The drawing under review shows one solid part. Ordinate dimensions are in mm from its lowest x, y, z. A direction names the side the tool comes from. Coordinates: 2 decimals unless noted, no trailing zeros. Loops run counter-clockwise (first coordinate to the right, second up) from the corner with the lowest first, then second, coordinate; pieces in that order, holes last. Notation, with made-up numbers: (57.25, -9) - (79.25, -9) arc R11 cw to (79.25, -4) - close; hole circle Ø6 at (86.25, 13). An arc over 180 degrees is marked (long way). Answer as a JSON object with one key per item and string values. Group by question number.
Item 1: We need section B-B (z = 12.75). Give the boundary of the cut face in (x, y).
Item 2: We need section A-A (x = 14.25). Give the boundary of the cut face in (y, z), then the cut area to 3 significant figures.
Item 3: We need section C-C (y = 44). Give the boundary of the cut face in (x, z), then the cut area to 3 significant figures.
Item 4: Tool access review of the marked faces 1, 2, 3 and 4: name each direction out of +Z, -Z, +X, -X, +Y, -Y from which nothing blocks a thin tool from reaching the whole face with its end or side.
Item 5: To check wall thickness, follow line 1 (Y direction, x = 2, z = 23); line 2 (Z direction, x = 6.5, y = 6.5); line 3 (Z direction, x = 6, y = 65.5). State the ranges of each line that lie inside material, in increasing order.
Item 6: We need section D-D (z = 6.25). Give the boundary of the cut face in (x, y).
Item 7: Clearance check with flat-ended pins moving along their axes: pin 1 (10 mm diameter, centred on x = 16.5, y = 45.5, fed in from -Z); pin 2 (7.5 mm diameter, centred on y = 42, z = 18, fed in from -X); pin 3 (7.5 mm diameter, centred on y = 42.5, z = 16.5, fed in from +X); pin 4 (5 mm diameter, centred on x = 21.5, y = 53.5, fed in from +Z). State where each tip first meets the part, or that it passes through.
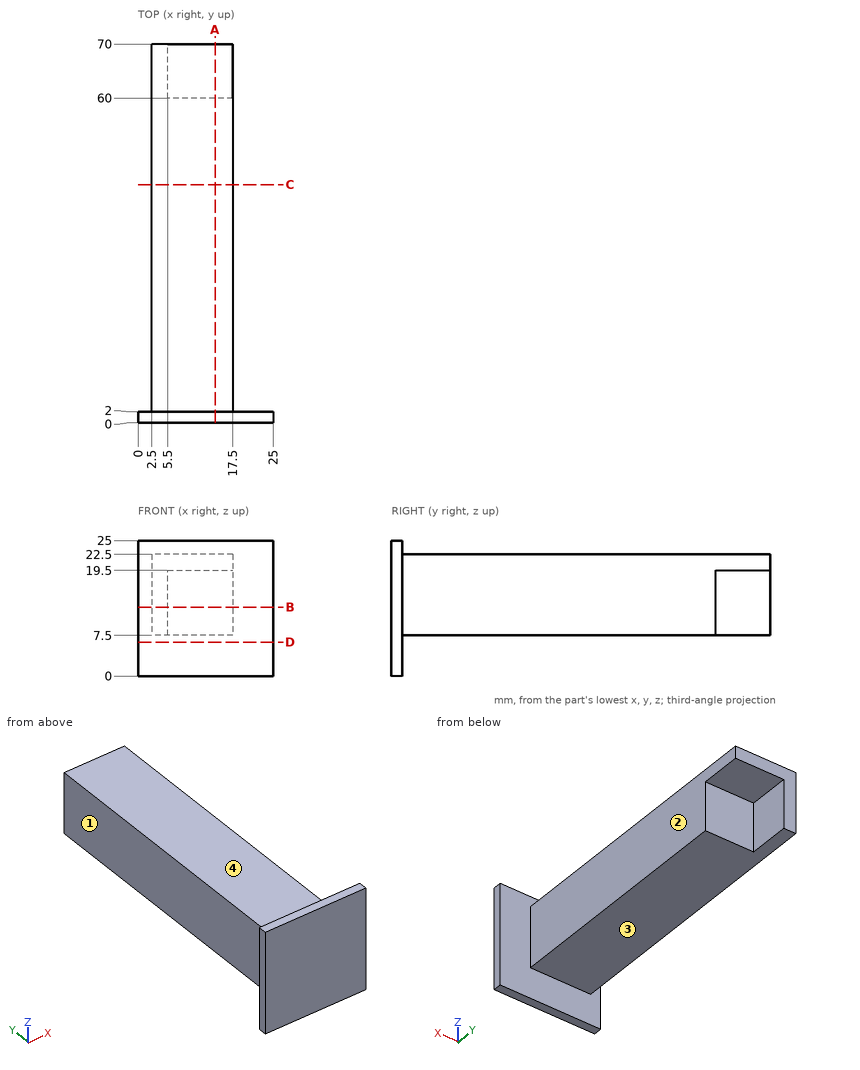
Check sheet entries:
{
 "1": {"outline": "(0, 0) - (25, 0) - (25, 2) - (17.5, 2) - (17.5, 60) - (5.5, 60) - (5.5, 70) - (2.5, 70) - (2.5, 2) - (0, 2) - close"},
 "2": {"outline": "(0, 0) - (2, 0) - (2, 7.5) - (60, 7.5) - (60, 19.5) - (70, 19.5) - (70, 22.5) - (2, 22.5) - (2, 25) - (0, 25) - close", "area": "950 mm2"},
 "3": {"outline": "(2.5, 7.5) - (17.5, 7.5) - (17.5, 22.5) - (2.5, 22.5) - close", "area": "225 mm2"},
 "4": {"face 1": "+Z, -Z, -X, +Y", "face 2": "+Z, -Z, +X, +Y", "face 3": "-Z, +X, -X, +Y", "face 4": "+Z, +X, -X, +Y"},
 "5": {"line 1": "y = 0 to 2", "line 2": "z = 7.5 to 22.5", "line 3": "z = 19.5 to 22.5"},
 "6": {"outline": "(0, 0) - (25, 0) - (25, 2) - (0, 2) - close"},
 "7": {"pin 1": "stops at z = 7.5", "pin 2": "stops at x = 2.5", "pin 3": "stops at x = 17.5", "pin 4": "passes through"}
}
